Autodesk Inventor part; units mm, degrees
ref_plane "YZ Plane" through (0, 0, 0) normal (1, 0, 0) x (0, 1, 0)
ref_plane "XZ Plane" through (0, 0, 0) normal (0, 1, 0) x (-1, 0, 0)
ref_plane "XY Plane" through (0, 0, 0) normal (0, 0, 1) x (1, 0, 0)
sketch "Sketch5" plane through (0, 0, 0) normal (0, 0, 1) x (1, 0, 0)
  line L0 (-70.25, 52) -> (70.25, 52)
  line L1 (70.25, 52) -> (70.25, -52)
  line L2 (70.25, -52) -> (-70.25, -52)
  line L3 (-70.25, -52) -> (-70.25, 52)
  point P0 (0, 0)
  point P1 (0, 52)
  point P2 (70.25, 0)
  dimension "d8" = 140.5
  dimension "d9" = 104
extrude "Extrusion5" add sketch "Sketch5" along normal blind 4
sketch "Sketch6" plane through (0, 0, 4) normal (0, 0, 1) x (1, 0, 0)
  circle A0 centre (-62.75, 35) radius 3
  circle A1 centre (-62.75, -35) radius 3
  circle A2 centre (62.75, 35) radius 3
  circle A3 centre (62.75, -35) radius 3
  line L0 (-70.25, 52) -> (-70.25, -52)
  line L1 (-70.25, -52) -> (70.25, -52)
  point P0 (0, 0)
  point P1 (0, 0)
  point P2 (0, -52)
  point P3 (-70.25, 0)
  dimension "d19" = 125.5
  dimension "d20" = 62.75
  dimension "d21" = 70
  dimension "d22" = 35
  dimension "d23" = 6
hole "Hole1" at (-62.75, 35, 4) at (62.75, 35, 4) at (62.75, -35, 4) at (-62.75, -35, 4) direction (0, 0, -1) diameter 5.5 end through all countersink diameter 11 countersink angle 90
chamfer "Chamfer1" distance 2 angle 45 4 edges at (70.25, -52, 2) (70.25, 52, 2) (-70.25, 52, 2) (-70.25, -52, 2)
properties part number "BC-10023" material "Alumínio 7075"
Verification items for the finished model (mm, model axes). Coordinates: 2 decimals unless noted, no trailing zeros. Loops run counter-clockwise (first coordinate to the right, second up) from the corner with the lowest first, then second, coordinate; pieces in that order, holes last. Notation, with made-up numbers: (37.25, 44) -> (81.25, 44) arc R33 cw to (81.25, 78) -> close; hole circle Ø6 at (72, 16.25). An arc over 180 degrees is marked (long way). Put each result on its own line as item: value.
1. Mould release check, pull along X, two halves, no side actions. Record for faces 1 (the face through (70.25, 1, 2)), 2 (the face through (60, -35, 1)), 3 (the face through (65.647, 35.38, 1.422)), 4 (the face through (-1, 1, 0)): pulls with the +X half, pulls with the -X half, needs draft (parallel to the pull), parting line crosses it, or undercut.
Result set:
face 1: pulls with the +X half
face 2: undercut
face 3: undercut
face 4: needs draft
2. Section check A-A, the plane x = -62.75. Record the boundary of the cut face in (y, z), then the cut area to 3 significant figures.
Result set:
outline: (-52, 0) -> (-37.75, 0) -> (-37.75, 1.25) -> (-40.5, 4) -> (-52, 4) -> close; (-32.25, 0) -> (32.25, 0) -> (32.25, 1.25) -> (29.5, 4) -> (-29.5, 4) -> (-32.25, 1.25) -> close; (37.75, 0) -> (52, 0) -> (52, 4) -> (40.5, 4) -> (37.75, 1.25) -> close
area: 357 mm^2
3. Thickness scan on line 1 (Y direction, x = 62.75, z = 0.8); line 2 (X direction, y = 35, z = 0.5); line 3 (X direction, y = -34.5, z = 3.7). Record the ranges inside material, lowest first.
Result set:
line 1: y = -52 to -37.75, -32.25 to 32.25, 37.75 to 52
line 2: x = -70.25 to -65.5, -60 to 60, 65.5 to 70.25
line 3: x = -70.25 to -67.93, -57.57 to 57.57, 67.93 to 70.25
4. Section check B-B, the plane y = 35. Record the boundary of the cut face in (x, z), then the cut area to 3 significant figures.
Result set:
outline: (-70.25, 0) -> (-65.5, 0) -> (-65.5, 1.25) -> (-68.25, 4) -> (-70.25, 4) -> close; (-60, 0) -> (60, 0) -> (60, 1.25) -> (57.25, 4) -> (-57.25, 4) -> (-60, 1.25) -> close; (65.5, 0) -> (70.25, 0) -> (70.25, 4) -> (68.25, 4) -> (65.5, 1.25) -> close
area: 503 mm^2
5. Gauge pin test, flat end, axial feed: P1, Ø4.5, axis at x = -62.75, y = 35, coming from the +Z side. Record the tip position at first contact, or that the pin passes through.
Result set:
P1: passes through
